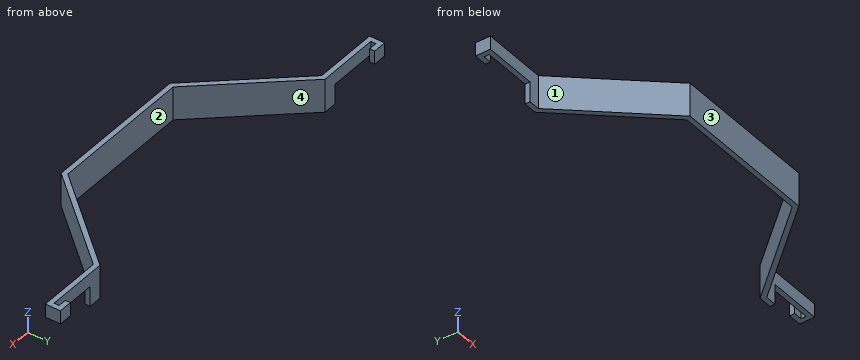
from build123d import *

# Parameters (mm, degrees)
BOSS_EXTRUDE1_DEPTH = 20
SKETCH2_W           = 32
SKETCH2_H           = 24
CUT_EXTRUDE1_DEPTH  = 190.205374127


with BuildPart() as part:
    # Sketch1 → Boss-Extrude1 (new body)
    with BuildSketch(Plane.XY):
        Polygon((-173.925616004, 29.588970737), (-136.925616004, 29.588970737), (-88.675616004, -25.411029263), (-3.675616004, -25.411029263), (44.574383996, 29.588970737), (81.574383996, 29.588970737), (81.574383996, 32.588970737), (76.574383996, 32.588970737), (76.574383996, 35.588970737), (84.574383996, 35.588970737), (84.574383996, 26.588970737), (45.933363597, 26.588970737), (-2.316636403, -28.411029263), (-90.034595605, -28.411029263), (-138.284595605, 26.588970737), (-176.925616004, 26.588970737), (-176.925616004, 35.588970737), (-168.925616004, 35.588970737), (-168.925616004, 32.588970737), (-173.925616004, 32.588970737), align=None)
    extrude(amount=BOSS_EXTRUDE1_DEPTH)

    # Sketch2 → Cut-Extrude1 (cut, through all)
    with BuildSketch(Plane(origin=(0, 35.588970737, 0), x_dir=(1, 0, 0), z_dir=(0, 1, 0))):
        with Locations((-160.925616004, 0)):
            Rectangle(SKETCH2_W, SKETCH2_H)
        with Locations((68.574383996, 0)):
            Rectangle(SKETCH2_W, SKETCH2_H)
    extrude(amount=-CUT_EXTRUDE1_DEPTH, mode=Mode.SUBTRACT)


solid = part.part
Model file for the job. Use its own axes, mm. Face numbers are marked on the shaded views. Give positions to 0.01 mm unless a question says otherwise; leave off trailing zeros. Loops run counter-clockwise (first coordinate to the right, second up) from the corner with the lowest first, then second, coordinate; pieces in that order, holes last. Notation, with made-up numbers: (11, 83) -> (47, 83) arc R25 ccw to (47, 97) -> close; hole circle Ø9 at (47.25, 80). An arc over 180 degrees is marked (long way). Use a Markdown table: item, result. Add a question column.
(1) Mould opens along X. For the marked faces 1, 2, 3 and 4 say: +X half, -X half, draft (parallel to the pull), parting line (faces both ways), or undercut.
(2) Wall check: line 1 along X through (y, z) = (4, 6.5); line 2 along X through (y, z) = (-9, 10.25); line 3 along Y through (x, z) = (-23, 9.5). Give the ranges that are in metal, low to high.
(3) Slice it at C-C on x = -42. List the corners of the cut face in (y, z).
(4) Slice it at B-B on z = 6. List the corners of the cut face in (x, y), and give its area (3 significant figures).
(5) Slice it at D-D on z = 17.5. List the corners of the cut face in (x, y), and give its area (4 significant figures).
(6) Drop flat-ended pins along their axis: pin 1 Ø4.5 at (x, y) = (75, 31.5) entering from -Z; pin 2 Ø1 at (x, z) = (-142.5, 15.5) entering from +Y; pin 3 Ø2 at (x, z) = (37, 3) entering from +Y. Give the stop position or say it passes through.
(7) Slice it at A-A on y = 18. List the corners of the cut face in (x, z).
Filled sheet:
| question | item | result |
|---|---|---|
| 1 | face 1 | -X half |
| 1 | face 2 | undercut |
| 1 | face 3 | draft |
| 1 | face 4 | undercut |
| 2 | line 1 | -118.47 to -114.48, 22.13 to 26.12 |
| 2 | line 2 | -107.06 to -103.07, 10.72 to 14.71 |
| 2 | line 3 | -28.41 to -25.41 |
| 3 | outline | (-28.41, 0) -> (-25.41, 0) -> (-25.41, 20) -> (-28.41, 20) -> close |
| 4 | outline | (-144.93, 26.59) -> (-138.28, 26.59) -> (-90.03, -28.41) -> (-2.32, -28.41) -> (45.93, 26.59) -> (52.57, 26.59) -> (52.57, 29.59) -> (44.57, 29.59) -> (-3.68, -25.41) -> (-88.68, -25.41) -> (-136.93, 29.59) -> (-144.93, 29.59) -> close |
| 4 | area | 742 mm2 |
| 5 | outline | (-176.93, 26.59) -> (-138.28, 26.59) -> (-90.03, -28.41) -> (-2.32, -28.41) -> (45.93, 26.59) -> (84.57, 26.59) -> (84.57, 35.59) -> (76.57, 35.59) -> (76.57, 32.59) -> (81.57, 32.59) -> (81.57, 29.59) -> (44.57, 29.59) -> (-3.68, -25.41) -> (-88.68, -25.41) -> (-136.93, 29.59) -> (-173.93, 29.59) -> (-173.93, 32.59) -> (-168.93, 32.59) -> (-168.93, 35.59) -> (-176.93, 35.59) -> close |
| 5 | area | 1,000 mm2 |
| 6 | pin 1 | z = 12 |
| 6 | pin 2 | y = 29.59 |
| 6 | pin 3 | y = 22.09 |
| 7 | outline | (-130.75, 0) -> (-126.76, 0) -> (-126.76, 20) -> (-130.75, 20) -> close; (34.41, 0) -> (38.4, 0) -> (38.4, 20) -> (34.41, 20) -> close |
